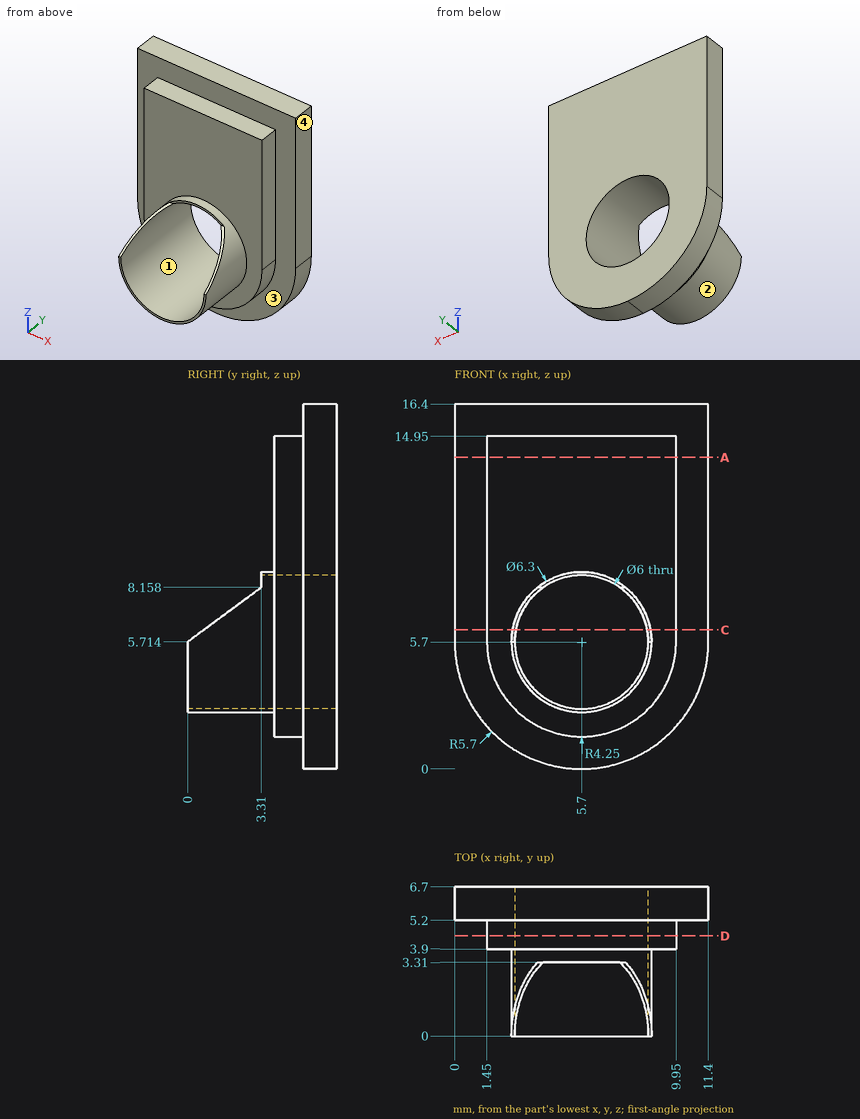
Could you check a few things on this drawing? It's one solid part, dimensions in mm from its lowest x, y, z. Give positions to 0.01 mm unless a question says otherwise; leave off trailing zeros. Order: outer loops, then holes, each group sorted by start corner. A loop starts at its lowest first (then second) coordinate and runs counter-clockwise, first axis right, second up. Notation, with made-up numbers: (30, -39.75) -> (50, -39.75) arc R17 ccw to (50, -26.75) -> close; hole circle Ø7 at (-38.75, 41.5). An arc over 180 degrees is marked (long way). Answer in a Markdown table with one row per item. Add a question column.
Item 1: We'd pull the mould along X, two halves only. Please class the marked faces 1, 2, 3 and 4: pulls with the +X half, pulls with the -X half, needs draft (parallel to the pull), parting line crosses it, or undercut.
Item 2: Imagine slicing it at C-C (z = 6.25). List the corners of the cut face in (x, y) for me.
Item 3: Imagine slicing it at A-A (z = 14). List the corners of the cut face in (x, y) for me.
Item 4: I'm going to push flat-ended pins straight in: P1, Ø0.7, axis at y = 4.5, z = 9, coming from the +X side; P2, Ø5.5, axis at x = 7.5, z = 11.5, coming from the -Y side; P3, Ø0.7, axis at x = 6, y = 4.5, coming from the +Z side. Where does each tip first touch, or does it pass through?
Item 5: Please list where these lines run through material, in increasing order: probe 1 along Z at (x, y) = (5.75, 5.5); probe 2 along Y at (x, z) = (1.25, 10); probe 3 along Y at (x, z) = (7.5, 14).
Item 6: Imagine slicing it at D-D (y = 4.5). List the corners of the cut face in (x, z) for me.
Result:
| question | item | result |
|---|---|---|
| 1 | face 1 | undercut |
| 1 | face 2 | parting line crosses it |
| 1 | face 3 | needs draft |
| 1 | face 4 | pulls with the +X half |
| 2 | outline | (0, 5.2) -> (1.45, 5.2) -> (1.45, 3.9) -> (2.6, 3.9) -> (2.6, 0.73) -> (2.75, 0.73) -> (2.75, 6.7) -> (0, 6.7) -> close; (8.65, 0.73) -> (8.8, 0.73) -> (8.8, 3.9) -> (9.95, 3.9) -> (9.95, 5.2) -> (11.4, 5.2) -> (11.4, 6.7) -> (8.65, 6.7) -> close |
| 3 | outline | (0, 5.2) -> (1.45, 5.2) -> (1.45, 3.9) -> (9.95, 3.9) -> (9.95, 5.2) -> (11.4, 5.2) -> (11.4, 6.7) -> (0, 6.7) -> close |
| 4 | P1 | x = 9.95 |
| 4 | P2 | y = 3.9 |
| 4 | P3 | z = 14.95 |
| 5 | probe 1 | 0 to 2.7, 8.7 to 16.4 |
| 5 | probe 2 | 5.2 to 6.7 |
| 5 | probe 3 | 3.9 to 6.7 |
| 6 | outline | (1.45, 5.7) arc R4.25 ccw to (9.95, 5.7) -> (9.95, 14.95) -> (1.45, 14.95) -> close; hole circle Ø6 at (5.7, 5.7) |
